The drawing under review shows one solid part. Ordinate dimensions are in mm from its lowest x, y, z. Give positions to 0.01 mm unless a question says otherwise; leave off trailing zeros. Write each loop counter-clockwise with the first axis right and the second up, starting at its lowest first coordinate (ties: lowest second). Pieces come first, ordered by that corner, then holes. Notation, with made-up numbers: (74.25, 61.25) - (104.25, 61.25) arc R16 cw to (104.25, 84.25) - close; hole circle Ø1 at (72, 86.5). An arc over 180 degrees is marked (long way). Write each question's results on one line, items separated by ' | '. Start each with the question number.
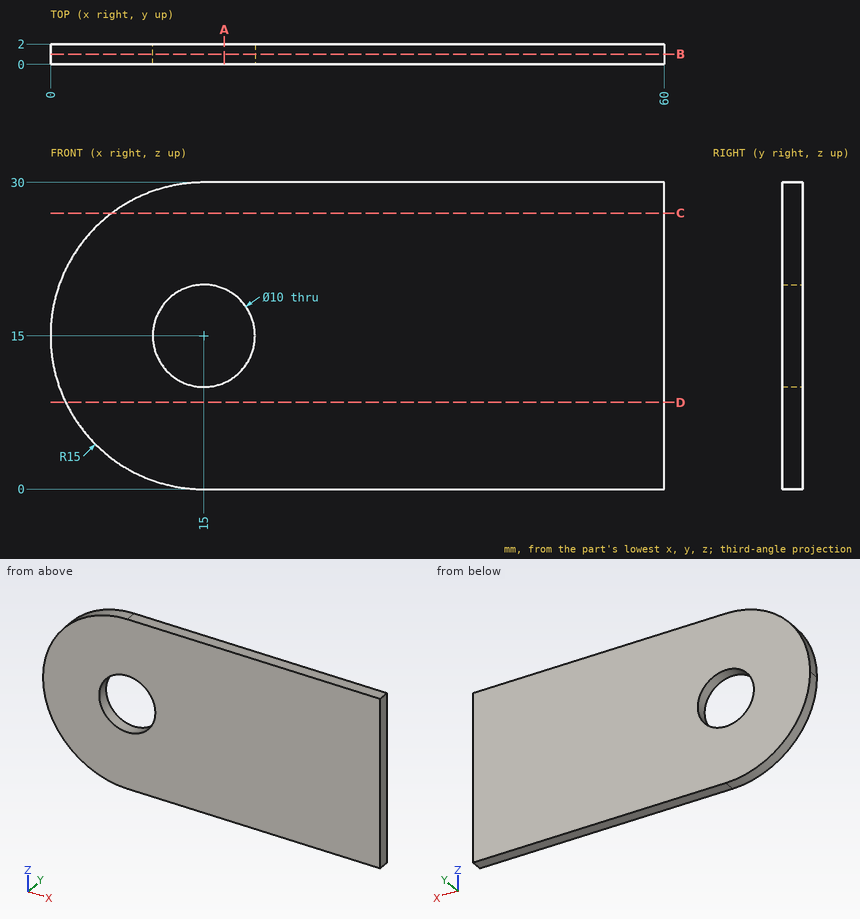
Q1. Add section D-D on z = 8.5. State the section outline as (x, y) points.
Q2. Add section B-B on y = 1. State the section outline as (x, z) points.
Q3. Add section A-A on x = 17. State the section outline as (y, z) points.
Q4. Add section C-C on z = 27. State the section outline as (x, y) points.
Q5. For line 1 along X through (y, z) = (1, 12.5); line 2 along X through (y, z) = (1.3, 11); line 3 along X through (y, z) = (1.5, 8), list the stretches that pass through material, from the lowest coordinate up. Write a range as [from, to].
Result:
1) outline: (1.48, 0) - (60, 0) - (60, 2) - (1.48, 2) - close
2) outline: (0, 15) arc R15 ccw to (15, 0) - (60, 0) - (60, 30) - (15, 30) arc R15 ccw to start; hole circle Ø10 at (15, 15)
3) outline: (0, 0) - (2, 0) - (2, 10.42) - (0, 10.42) - close; (0, 19.58) - (2, 19.58) - (2, 30) - (0, 30) - close
4) outline: (6, 0) - (60, 0) - (60, 2) - (6, 2) - close
5) line 1: x = [0.21, 10.67], [19.33, 60] | line 2: x = [0.54, 12], [18, 60] | line 3: x = [1.73, 60]
